from build123d import *

# Parameters (mm, degrees)
SKETCH1_W           = 53.47
SKETCH1_H           = 12.33
BASE_EXTRUDE_DEPTH  = 12.7
BOSS_EXTRUDE1_DEPTH = 6.07
SKETCH4_R           = 0.5
CUT_EXTRUDE1_DEPTH  = 5.08
SKETCH5_R           = 0.5
CUT_EXTRUDE2_DEPTH  = 5.08
SKETCH6_R           = 0.3556
BOSS_EXTRUDE2_DEPTH = 2.54
LPATTERN1_COUNT     = 13
LPATTERN1_PITCH     = 2.7686
LPATTERN2_COUNT     = 13
LPATTERN2_PITCH     = 2.7686
LPATTERN3_COUNT     = 12
LPATTERN3_PITCH     = 2.7686
SKETCH7_R           = 0.3556
BOSS_EXTRUDE3_DEPTH = 2.54
LPATTERN4_COUNT     = 12
LPATTERN4_PITCH     = 2.7686
SKETCH12_R          = 1.304277921
BOSS_EXTRUDE4_DEPTH = 6.07
SKETCH9_W           = 6.35508
SKETCH9_H           = 10.16
CUT_EXTRUDE3_DEPTH  = 9.33
SKETCH11_R          = 1.4
CUT_EXTRUDE4_DEPTH  = 6.08


with BuildPart() as part:
    # Sketch1 → Base-Extrude (new body)
    with BuildSketch(Plane(origin=(0, 0, 0), x_dir=(1, 0, 0), z_dir=(0, 1, 0))):
        with Locations((16.575, 4.395)):
            Rectangle(SKETCH1_W, SKETCH1_H)
    extrude(amount=BASE_EXTRUDE_DEPTH)

    # Sketch2 → Boss-Extrude1 (add)
    with BuildSketch(Plane(origin=(0, 0, -10.56), x_dir=(-1, 0, 0), z_dir=(0, 0, -1))):
        with BuildLine():
            Line((-32.654431338, 2.286), (-0.495568662, 2.286))
            ThreePointArc((-0.495568662, 2.286), (1.120925043, 2.8667787), (1.998186376, 4.34352118))
            Line((1.998186376, 4.34352118), (2.538755038, 7.13752118))
            ThreePointArc((2.538755038, 7.13752118), (2.0042213, 9.236493705), (0.045, 10.16))
            Line((0.045, 10.16), (-33.195, 10.16))
            ThreePointArc((-33.195, 10.16), (-35.1542213, 9.236493705), (-35.688755038, 7.13752118))
            Line((-35.688755038, 7.13752118), (-35.148186376, 4.34352118))
            ThreePointArc((-35.148186376, 4.34352118), (-34.270925043, 2.8667787), (-32.654431338, 2.286))
        make_face()
    extrude(amount=BOSS_EXTRUDE1_DEPTH)

    # Sketch4 → Cut-Extrude1 (cut)
    with BuildSketch(Plane(origin=(0, 0, -16.63), x_dir=(-1, 0, 0), z_dir=(0, 0, -1))):
        with Locations((0, 7.62)):
            Circle(SKETCH4_R)
    cut_extrude1 = extrude(amount=-CUT_EXTRUDE1_DEPTH, mode=Mode.SUBTRACT)

    # Sketch5 → Cut-Extrude2 (cut)
    with BuildSketch(Plane(origin=(0, 0, -16.63), x_dir=(-1, 0, 0), z_dir=(0, 0, -1))):
        with Locations((-1.397, 5.08)):
            Circle(SKETCH5_R)
    cut_extrude2 = extrude(amount=-CUT_EXTRUDE2_DEPTH, mode=Mode.SUBTRACT)

    # Sketch6 → Boss-Extrude2 (add)
    with BuildSketch(Plane.XZ):
        Circle(SKETCH6_R)
    boss_extrude2 = extrude(amount=BOSS_EXTRUDE2_DEPTH)

    # LPattern1: Boss-Extrude2 ×13
    with Locations(*[(i * LPATTERN1_PITCH, 0, 0) for i in range(1, LPATTERN1_COUNT)]):
        add(boss_extrude2)

    # LPattern2: Cut-Extrude1 ×13
    with Locations(*[(i * LPATTERN2_PITCH, 0, 0) for i in range(1, LPATTERN2_COUNT)]):
        add(cut_extrude1, mode=Mode.SUBTRACT)

    # LPattern3: Cut-Extrude2 ×12
    with Locations(*[(i * LPATTERN3_PITCH, 0, 0) for i in range(1, LPATTERN3_COUNT)]):
        add(cut_extrude2, mode=Mode.SUBTRACT)

    # Sketch7 → Boss-Extrude3 (add)
    with BuildSketch(Plane.XZ):
        with Locations((1.397, -2.54)):
            Circle(SKETCH7_R)
    boss_extrude3 = extrude(amount=BOSS_EXTRUDE3_DEPTH)

    # LPattern4: Boss-Extrude3 ×12
    with Locations(*[(i * LPATTERN4_PITCH, 0, 0) for i in range(1, LPATTERN4_COUNT)]):
        add(boss_extrude3)

    # Sketch12 → Boss-Extrude4 (add)
    with BuildSketch(Plane(origin=(0, 0, -10.56), x_dir=(-1, 0, 0), z_dir=(0, 0, -1))):
        Polygon((-41.595, 9.82), (-42.98, 7.421109632), (-41.595, 5.022219263), (-38.825, 5.022219263), (-37.44, 7.421109632), (-38.825, 9.82), align=None)
        with Locations((-40.21, 7.421109632)):
            Circle(SKETCH12_R, mode=Mode.SUBTRACT)
    boss_extrude4 = extrude(amount=BOSS_EXTRUDE4_DEPTH)

    # Sketch9 → Cut-Extrude3 (cut)
    with BuildSketch(Plane.XY.offset(1.77)):
        with Locations((-6.98246, 7.62)):
            Rectangle(SKETCH9_W, SKETCH9_H)
    cut_extrude3 = extrude(amount=-CUT_EXTRUDE3_DEPTH, mode=Mode.SUBTRACT)

    # Sketch11 → Cut-Extrude4 (cut, through all)
    with BuildSketch(Plane(origin=(0, 2.54, 0), x_dir=(-1, 0, 0), z_dir=(0, 1, 0))):
        with Locations((7.06, -1.27)):
            Circle(SKETCH11_R)
    cut_extrude4 = extrude(amount=-CUT_EXTRUDE4_DEPTH, mode=Mode.SUBTRACT)

    # Mirror1: Boss-Extrude4, Cut-Extrude3, Cut-Extrude4 across plane
    add(boss_extrude4.mirror(Plane(origin=(16.575, 0, 0), x_dir=(0, 0, 1), z_dir=(1, 0, 0))))
    add(cut_extrude3.mirror(Plane(origin=(16.575, 0, 0), x_dir=(0, 0, 1), z_dir=(1, 0, 0))), mode=Mode.SUBTRACT)
    add(cut_extrude4.mirror(Plane(origin=(16.575, 0, 0), x_dir=(0, 0, 1), z_dir=(1, 0, 0))), mode=Mode.SUBTRACT)


solid = part.part
Input: part model. Units: mm. Frame: model coordinates. A direction names the side the tool comes from. Give positions to 0.01 mm unless a question says otherwise; leave off trailing zeros. Write each loop counter-clockwise with the first axis right and the second up, starting at its lowest first coordinate (ties: lowest second). Pieces come first, ordered by that corner, then holes.
Q1. Material intervals for probe 1 along X at (y, z) = (5.75, -13.5); probe 2 along Y at (x, z) = (38, -6.5); probe 3 along Y at (x, z) = (33, 0.75), sorted ascending.
Q2. Section B-B, the plane x = 40.21. Output: boundary loops of the cut face in (y, z).
Q3. Section D-D, the plane z = -4. Output: boundary loops of the cut face in (x, y), plus the area to 3 significant figures.
Q4. First-contact query: P1, Ø0.8, axis at x = 19, y = 7.5, coming from the -Z side; P2, Ø3, axis at x = 20.5, z = -15, coming from the -Y side; P3, Ø1, axis at y = 10, z = -1, coming from the +X side; P4, Ø1.8, axis at x = 9, z = -13, coming from the +Y side. Flat tips, straight axial feed; report the tip coordinate or a pass-through.
Q5. Section A-A, the plane y = -1.5. State how many separate pieces and enclosed holes the cut face has, plus the area to 3 significant figures.
Q6. Pull-direction query (X, two-part tool) for faces 4 (the face through (21, 5, -11.55)), 5 (the face through (17, 2.286, -14)), 6 (the face through (-9.128, 8.637, -13.553)); classes: pulls with the +X half, pulls with the -X half, needs draft (parallel to the pull), parting line crosses it, or undercut.
Q7. Set-up query: faces 1 (the face through (40, 9.82, -14)), 2 (the face through (-4.992, 6.205, -13.553)), 3 (the face through (24.045, 5.102, -14.126)). Return all of +Z, -Z, +X, -X, +Y, -Y with unobstructed straight access to the full face (end or side cutting, diameter ignored); none if empty.
Filled in:
1. probe 1: x = -8.87 to -5.25, -2.27 to 35.42, 38.4 to 42.02
1. probe 2: y = 0 to 2.54
1. probe 3: y = 0 to 12.7
2. outline: (0, -10.56) - (5.02, -10.56) - (5.02, -16.63) - (6.12, -16.63) - (6.12, -10.56) - (8.73, -10.56) - (8.73, -16.63) - (9.82, -16.63) - (9.82, -10.56) - (12.7, -10.56) - (12.7, -7.56) - (2.54, -7.56) - (2.54, -2.67) - (0, -2.67) - close; (0, 0.13) - (2.54, 0.13) - (2.54, 1.77) - (0, 1.77) - close
3. outline: (-10.16, 0) - (43.31, 0) - (43.31, 2.54) - (36.95, 2.54) - (36.95, 12.7) - (-3.8, 12.7) - (-3.8, 2.54) - (-10.16, 2.54) - close
3. area: 550 mm2
4. P1: stops at z = -16.63
4. P2: stops at y = 2.29
4. P3: stops at x = 36.95
4. P4: stops at y = 10.16
5. separate pieces: 25
5. enclosed holes: 0
5. area: 9.93 mm2
6. face 4: undercut
6. face 5: needs draft
6. face 6: pulls with the -X half
7. face 1: -Z, +X, +Y
7. face 2: -Z, -Y
7. face 3: -Z
